Geometry check sheet. Reference: the model listing, model coordinates, mm. Face numbers are marked on the shaded views. A direction names the side the tool comes from. Round coordinates to 2 decimals unless told otherwise and drop trailing zeros. Write each loop counter-clockwise with the first axis right and the second up, starting at its lowest first coordinate (ties: lowest second). Pieces come first, ordered by that corner, then holes. Notation, with made-up numbers: M 87.5,85 L 111.5,85 A29 ccw 111.5,105 Z; hole C -35,83.25 d4. An arc over 180 degrees is marked long. One line per item, written item: value. Start each with the question number.
1. Release check for a two-part mould opening along X. For the marked faces 1, 2, 3 and 4 record: pulls with the +X half, pulls with the -X half, needs draft (parallel to the pull), parting line crosses it, or undercut.
2. Depth check by flat-ended pin: P1, Ø5, axis at x = -5, z = 4, coming from the -Y side (3 decimals); P2, Ø3.5, axis at y = -4.5, z = 3, coming from the +X side; P3, Ø12, axis at y = 8.5, z = -10.5, coming from the -X side. Enter the tip coordinate at first touch or a pass-through.
3. Access from +Z, -Z, +X, -X, +Y, -Y to the whole of each face (thin tool, end or side, straight path). Record for the marked faces 5, 6, 7, 8 and 9.
4. Section check D-D (x = -5.5). Record the boundary of the cut face in (y, z) (1 decimal), and give its area (3 significant figures).
5. Section check B-B (z = 2.5). Record the boundary of the cut face in (x, y) (1 decimal), and give its area (3 significant figures).
6. Section check C-C (y = 8.25). Record the boundary of the cut face in (x, z), and give its area (3 significant figures).
7. Section check A-A (x = 0.5). Record the boundary of the cut face in (y, z) (1 decimal).
8. Scan lines: probe 1 along X at (y, z) = (-3.75, 6); probe 2 along Z at (x, y) = (6.25, 7.25); probe 3 along Y at (x, z) = (-1.25, -10.5) (3 decimals). Record each from-to range of solid material in increasing order. Write a range as [from, to].
Autodesk Fusion 360 part; units mm, degrees
sketch "Sketch1" plane through (0, 0, 0) normal (0, 1, 0) x (1, 0, 0)
  line L0 (10.9855, 12.8905) -> (-10.9855, 12.8905)
  line L1 (-10.9855, 12.8905) -> (-10.9855, -12.8905)
  line L2 (-10.9855, -12.8905) -> (10.9855, -12.8905)
  line L3 (10.9855, -12.8905) -> (10.9855, 12.8905)
  line L4 (10.9855, 12.8905) -> (-10.9855, -12.8905) construction
  line L5 (-10.9855, 12.8905) -> (10.9855, -12.8905) construction
  dimension "d1" = 21.971
  dimension "d2" = 25.781
extrude "Extrude1" add sketch "Sketch1" along normal blind 19.2786
sketch "Sketch2" plane through (0, 0, 0) normal (0, -1, 0) x (1, 0, 0)
  line L0 (10.9855, -12.8905) -> (10.9855, 12.8905)
  line L1 (10.9855, 12.8905) -> (-10.9855, 12.8905)
  line L2 (-10.9855, 12.8905) -> (-10.9855, -12.8905)
  line L3 (-10.9855, -12.8905) -> (10.9855, -12.8905)
  line L4 (12.192, -15.621) -> (-12.192, -15.621)
  line L5 (-12.192, -15.621) -> (-12.192, 15.621)
  line L6 (-12.192, 15.621) -> (12.192, 15.621)
  line L7 (12.192, 15.621) -> (12.192, -15.621)
  line L8 (12.192, -15.621) -> (-12.192, 15.621) construction
  line L9 (-12.192, -15.621) -> (12.192, 15.621) construction
  dimension "d5" = 24.384
  dimension "d6" = 31.242
extrude "Extrude2" add sketch "Sketch2" along normal blind 1.905 contours L0 L1 L2 L3 | L4 L5 L6 L7
sketch "Sketch3" plane through (0, -1.905, 0) normal (0, -1, 0) x (1, 0, 0)
  line L0 (12.192, 15.621) -> (-12.192, 15.621)
  line L1 (-12.192, 15.621) -> (-12.192, -15.621)
  line L2 (-12.192, -15.621) -> (12.192, -15.621)
  line L3 (12.192, -15.621) -> (12.192, 15.621)
  line L4 (-9.779, 12.0142) -> (-1.8288, 12.0142)
  line L5 (-1.8288, 12.0142) -> (-1.8288, -12.0142)
  line L6 (-1.8288, -12.0142) -> (-9.779, -12.0142)
  line L7 (-9.779, -12.0142) -> (-9.779, 12.0142)
  dimension "d9" = 3.6068
  dimension "d10" = 3.6068
  dimension "d11" = 2.413
  dimension "d12" = 7.9502
ref_plane "WorkPlane1" through (-1.8288, -1.905, 0) normal (-1, 0, 0) x (0, 0, -1)
sketch "Sketch5" plane through (-1.8288, -1.905, 0) normal (-1, 0, 0) x (0, 1, 0)
  line L0 (0, -12.0142) -> (0, 12.0142)
  line L1 (0, 12.0142) -> (-4.3758, -7.048)
  arc A0 (-4.3758, -7.048) -> (0, -12.0142) centre (1.0537, -6.6748) ccw
  dimension "d14" = 19.558
extrude "Extrude3" add sketch "Sketch5" along normal blind 7.9502
mirror "Mirror1" about plane through (0, 0, 0) normal (1, 0, 0) of "Extrude3"
equation "d10 = d9"
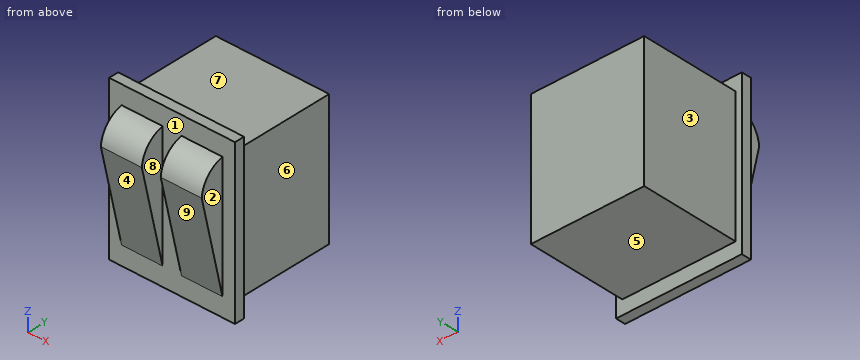
Result sheet:
1. face 1: undercut
1. face 2: pulls with the +X half
1. face 3: pulls with the -X half
1. face 4: needs draft
2. P1: stops at y = -6.155
2. P2: stops at x = 9.78
2. P3: stops at x = -10.99
3. face 5: -Z, +X, -X, +Y
3. face 6: +Z, -Z, +X, +Y
3. face 7: +Z, +X, -X, +Y
3. face 8: +Z, -Z, -Y
3. face 9: -Z, +X, -X, -Y
4. outline: M -6.3,7 L -1.9,-12 L -1.9,-15.6 L 0,-15.6 L 0,-12.9 L 19.3,-12.9 L 19.3,12.9 L 0,12.9 L 0,15.6 L -1.9,15.6 L -1.9,12 A5.4 ccw Z
4. area: 614 mm2
5. outline: M -12.2,-1.9 L -9.8,-1.9 L -9.8,-5.2 L -1.8,-5.2 L -1.8,-1.9 L 1.8,-1.9 L 1.8,-5.2 L 9.8,-5.2 L 9.8,-1.9 L 12.2,-1.9 L 12.2,0 L 11,0 L 11,19.3 L -11,19.3 L -11,0 L -12.2,0 Z
5. area: 523 mm2
6. outline: M -10.99,-12.89 L 10.99,-12.89 L 10.99,12.89 L -10.99,12.89 Z
6. area: 566 mm2
7. outline: M -1.9,-15.6 L 0,-15.6 L 0,-12.9 L 19.3,-12.9 L 19.3,12.9 L 0,12.9 L 0,15.6 L -1.9,15.6 Z
8. probe 1: x = [-9.78, -1.83], [1.83, 9.78]
8. probe 2: z = [-12.89, 12.89]
8. probe 3: y = [-1.905, 19.279]
